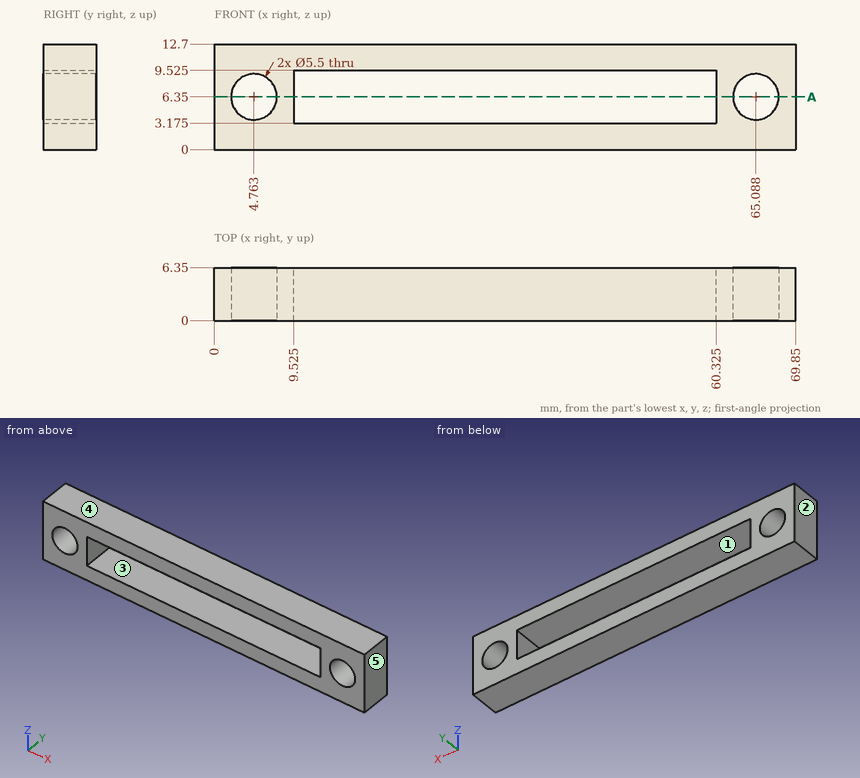
Drawing for the job (mm, zero at the part's lowest x, y, z). A direction names the side the tool comes from. Give positions to 0.01 mm unless a question says otherwise; leave off trailing zeros. Write item = value, one per line. Start each with the question number.
1) Pull direction Z, two halves, no side cores. Call the marked faces 3, 4 and 5: +Z half, -Z half, draft (parallel to the pull), parting line (faces both ways), or undercut.
2) Probe probe 1 along Z at (x, y) = (13.5, 4.75) (1 decimal); probe 2 along Z at (x, y) = (6, 3) (1 decimal). List the from-to ranges inside material, lowest first. Write a range as from..to.
3) Band-saw the part on A-A on z = 6.35. Count the separate pieces of the cut face and the enclosed holes in it.
4) Tool access for the marked faces 1 and 2: list every direction of +Z, -Z, +X, -X, +Y, -Y with a clear straight run to the whole face (end or side of a thin tool).
Final values:
q1.face_3 = undercut
q1.face_4 = +Z half
q1.face_5 = draft
q2.probe_1 = 0..3.2, 9.5..12.7
q2.probe_2 = 0..3.9, 8.8..12.7
q3.separate_pieces = 4
q3.enclosed_holes = 0
q4.face_1 = +Y, -Y
q4.face_2 = +Z, -Z, -X, +Y, -Y
